Verification items for the finished model (mm, model axes). A direction names the side the tool comes from. Round coordinates to 2 decimals unless told otherwise and drop trailing zeros. Loops run counter-clockwise (first coordinate to the right, second up) from the corner with the lowest first, then second, coordinate; pieces in that order, holes last. Notation, with made-up numbers: (81.25, 47) - (133.25, 47) arc R31 cw to (133.25, 80) - close; hole circle Ø1 at (70, 67). An arc over 180 degrees is marked (long way). Use CSV: the item, a comma, the result in double quotes.
```python
from build123d import *

# Parameters (mm, degrees)
SKETCH_1_W          = 37
SKETCH_1_H          = 57
EXTRUDE_1_DEPTH     = 2
SKETCH_2_W          = 3
SKETCH_2_H          = 57
EXTRUDE_2_DEPTH     = 19.5
SKETCH_3_W          = 2.5
SKETCH_3_H          = 8.5
EXTRUDE_3_DEPTH     = 19.5
SKETCH_4_R          = 1.55
CUT_EXTRUDE_1_DEPTH = 40.17588544
SKETCH_6_R          = 2.5
EXTRUDE_4_DEPTH     = 3
SKETCH_7_R          = 2.15
CUT_EXTRUDE_2_DEPTH = 3
FILLET_1_R          = 3
CHAMFER_2_SIZE      = 1


with BuildPart() as part:
    # 草图1 → 凸台-拉伸1 (new body)
    with BuildSketch(Plane.XY):
        Rectangle(SKETCH_1_W, SKETCH_1_H)
    extrude(amount=EXTRUDE_1_DEPTH)

    # 草图2 → 凸台-拉伸2 (add)
    with BuildSketch(Plane.XY.offset(2)):
        with Locations((-17, 0)):
            Rectangle(SKETCH_2_W, SKETCH_2_H)
    extrude(amount=EXTRUDE_2_DEPTH)

    # 草图3 → 凸台-拉伸3 (add)
    with BuildSketch(Plane.XY.offset(2)):
        with Locations((11.75, -24.25)):
            Rectangle(SKETCH_3_W, SKETCH_3_H)
        with Locations((11.75, 24.25)):
            Rectangle(SKETCH_3_W, SKETCH_3_H)
    extrude(amount=EXTRUDE_3_DEPTH)

    # 草图4 → 切除-拉伸1 (cut, through all)
    with BuildSketch(Plane.XY.offset(2)):
        with Locations((0, 5.6)):
            Circle(SKETCH_4_R)
        with Locations((0, -5.6)):
            Circle(SKETCH_4_R)
    extrude(amount=-CUT_EXTRUDE_1_DEPTH, mode=Mode.SUBTRACT)

    # 草图6 → 凸台-拉伸4 (add)
    with BuildSketch(Plane.ZY.offset(18.5)):
        with Locations(Location((11.5, -9.9, 0), (0, 0, 90))):
            Circle(SKETCH_6_R)
    extrude(amount=EXTRUDE_4_DEPTH)

    # 草图7 → 切除-拉伸2 (cut)
    with BuildSketch(Plane(origin=(13, 0, 0), x_dir=(0, 0, -1), z_dir=(1, 0, 0))):
        with Locations((-17, -23.793044535)):
            Circle(SKETCH_7_R)
        with Locations((-7, -23.793044535)):
            Circle(SKETCH_7_R)
        with Locations(Location((-7, 23.793044535, 0), (0, 0, 90))):
            Circle(SKETCH_7_R)
        with Locations(Location((-17, 23.793044535, 0), (0, 0, 90))):
            Circle(SKETCH_7_R)
    extrude(amount=-CUT_EXTRUDE_2_DEPTH, mode=Mode.SUBTRACT)

    # 圆角1
    fillet_1_edges = [part.edges().sort_by_distance(p)[0] for p in [
        (-17, -28.5, 21.5),
        (-17, 28.5, 21.5),
        (11.75, -28.5, 21.5),
        (11.75, -20, 21.5),
        (11.75, 20, 21.5),
        (11.75, 28.5, 21.5),
    ]]
    fillet(fillet_1_edges, radius=FILLET_1_R)

    # 倒角2
    chamfer_2_edges = [part.edges().sort_by_distance(p)[0] for p in [
        (10.5, -24.25, 2),
        (10.5, 24.25, 2),
    ]]
    chamfer(chamfer_2_edges, length=CHAMFER_2_SIZE)


solid = part.part
```
1) Cross-section at D-D, the plane z = 11.5. Record the cut outline in (x, y), then the cut area to 4 significant figures.
Returned:
outline,"(-21.5, -12.4) - (-18.5, -12.4) - (-18.5, -28.5) - (-15.5, -28.5) - (-15.5, 28.5) - (-18.5, 28.5) - (-18.5, -7.4) - (-21.5, -7.4) - close; (10.5, -28.5) - (13, -28.5) - (13, -20) - (10.5, -20) - close; (10.5, 20) - (13, 20) - (13, 28.5) - (10.5, 28.5) - close"
area,"228.5 mm²"
2) Gauge pin test, flat ends, axial feed: pin 1 Ø2.5 at (y, z) = (-25, 16) entering from +X; pin 2 Ø4 at (y, z) = (23.79, 17) entering from -X; pin 3 Ø17 at (x, y) = (-4.5, -5) entering from +Z. Record the tip position at first contact, or that the pin passes through.
Returned:
pin 1,"stops at x = 13"
pin 2,"stops at x = -18.5"
pin 3,"stops at z = 2"
3) Mould release check, pull along X, two halves, no side actions. Record for faces 1 (the face through (18.5, 0, 1)), 2 (the face through (11.768, 25.844, 7.646)), 3 (the face through (1, 0, 2)), 4 (the face through (10.5, 24, 12)): +X half, -X half, draft (parallel to the pull), parting line (faces both ways), or undercut.
Returned:
face 1,"+X half"
face 2,"draft"
face 3,"undercut"
face 4,"undercut"
4) Cross-section at B-B, the plane z = 7. Record the cut outline in (x, y).
Returned:
outline,"(-18.5, -28.5) - (-15.5, -28.5) - (-15.5, 28.5) - (-18.5, 28.5) - close; (10.5, -28.5) - (13, -28.5) - (13, -25.94) - (10.5, -25.94) - close; (10.5, -21.64) - (13, -21.64) - (13, -20) - (10.5, -20) - close; (10.5, 20) - (13, 20) - (13, 21.64) - (10.5, 21.64) - close; (10.5, 25.94) - (13, 25.94) - (13, 28.5) - (10.5, 28.5) - close"
5) Cross-section at C-C, the plane x = 0. Record the cut outline in (y, z), then the cut area to 3 significant figures.
Returned:
outline,"(-28.5, 0) - (-7.15, 0) - (-7.15, 2) - (-28.5, 2) - close; (-4.05, 0) - (4.05, 0) - (4.05, 2) - (-4.05, 2) - close; (7.15, 0) - (28.5, 0) - (28.5, 2) - (7.15, 2) - close"
area,"102 mm²"
6) Thickness scan on probe 1 along Y at (x, z) = (0, 0.45); probe 2 along X at (y, z) = (5.5, 1.75); probe 3 along Y at (x, z) = (12, 6.75). Record the ranges inside material, lowest first. Write a range as [from, to].
Returned:
probe 1,"y = [-28.5, -7.15], [-4.05, 4.05], [7.15, 28.5]"
probe 2,"x = [-18.5, -1.55], [1.55, 18.5]"
probe 3,"y = [-28.5, -25.93], [-21.66, -20], [20, 21.66], [25.93, 28.5]"
7) Cross-section at A-A, the plane y = 5.6. Record the cut outline in (x, z), then the cut area to 3 significant figures.
Returned:
outline,"(-18.5, 0) - (-1.55, 0) - (-1.55, 2) - (-15.5, 2) - (-15.5, 21.5) - (-18.5, 21.5) - close; (1.55, 0) - (18.5, 0) - (18.5, 2) - (1.55, 2) - close"
area,"126 mm²"
8) Access from +Z, -Z, +X, -X, +Y, -Y to the whole of each face (thin tool, end or side, straight path). Record for faces 5 (the face through (11.77, -20.9, 20.64)), 6 (the face through (-15.5, 0, 12)), 7 (the face through (11.768, -21.98, 5.844)), 8 (the face through (-20, -10, 14)).
Returned:
face 5,"+Z, +X"
face 6,"+Z, +Y, -Y"
face 7,"+X"
face 8,"-X"
